CAD build for the part. Positions are in the model's coordinates, mm. Round coordinates to 2 decimals unless told otherwise and drop trailing zeros. Loops run counter-clockwise (first coordinate to the right, second up) from the corner with the lowest first, then second, coordinate; pieces in that order, holes last. Notation, with made-up numbers: M -24.75,41.5 L -8.75,41.5 A6 cw -8.75,46.5 Z; hole C 72.5,72 d10. An arc over 180 degrees is marked long. Use one line per item in the form item = value.
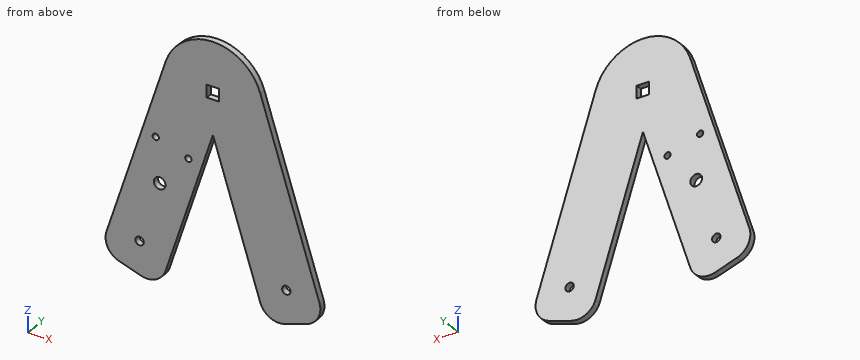
from build123d import *

# Parameters (mm, degrees)
SKETCH1_R           = 2.15
SKETCH1_R_2         = 3
SKETCH1_R_3         = 1.6
SKETCH1_W           = 6.35
SKETCH1_H           = 6.35
BOSS_EXTRUDE1_DEPTH = 3.175
FILLET1_R           = 10


with BuildPart() as part:
    # Sketch1 → Boss-Extrude1 (new body)
    with BuildSketch(Plane(origin=(0, 0, 0), x_dir=(1, 0, 0), z_dir=(0, 1, 0))):
        with BuildLine():
            Line((-57.479624947, 95.534974299), (-24.175240451, -7.792159464))
            ThreePointArc((-24.175240451, -7.792159464), (0, -25.4), (24.175240451, -7.792159464))
            Line((24.175240451, -7.792159464), (57.479624947, 95.534974299))
            Line((57.479624947, 95.534974299), (27.260574383, 105.27517363))
            Line((27.260574383, 105.27517363), (0, 20.69901171))
            Line((0, 20.69901171), (-27.260574383, 105.27517363))
            Line((-27.260574383, 105.27517363), (-57.479624947, 95.534974299))
        make_face()
        with Locations((37.5, 85.295548682)):
            Circle(SKETCH1_R, mode=Mode.SUBTRACT)
        with Locations((-37.5, 85.295548682)):
            Circle(SKETCH1_R, mode=Mode.SUBTRACT)
        with Locations((-27.222939289, 53.410881158)):
            Circle(SKETCH1_R_2, mode=Mode.SUBTRACT)
        with Locations((-29.231398698, 31.119883181)):
            Circle(SKETCH1_R_3, mode=Mode.SUBTRACT)
        with Locations((-12.575229096, 36.488496985)):
            Circle(SKETCH1_R_3, mode=Mode.SUBTRACT)
        Rectangle(SKETCH1_W, SKETCH1_H, mode=Mode.SUBTRACT)
    extrude(amount=BOSS_EXTRUDE1_DEPTH)

    # Fillet1
    fillet1_edges = [part.edges().sort_by_distance(p)[0] for p in [
        (-27.260574383, 1.5875, -105.27517363),
        (27.260574383, 1.5875, -105.27517363),
        (57.479624947, 1.5875, -95.534974299),
        (-57.479624947, 1.5875, -95.534974299),
    ]]
    fillet(fillet1_edges, radius=FILLET1_R)


solid = part.part
1. Cut at A-A on z = -70. Write the cut outline in (x, y) (3 decimals), and give its area (3 significant figures).
Completed:
outline = M -49.249,0 L -15.891,0 L -15.891,3.175 L -49.249,3.175 Z; M 15.891,0 L 49.249,0 L 49.249,3.175 L 15.891,3.175 Z
area = 212 mm2
2. Cut at B-B on y = 1.2. State how many separate pieces and enclosed holes the cut face has, and give its area (3 significant figures).
Completed:
separate_pieces = 1
enclosed_holes = 6
area = 7,380 mm2
3. Cut at C-C on x = 17. Write the cut outline in (y, z) (3 decimals), and give its area (3 significant figures).
Completed:
outline = M 0,-73.442 L 3.175,-73.442 L 3.175,18.872 L 0,18.872 Z
area = 293 mm2
4. Cut at D-D on x = -45. Write the cut outline in (y, z) (3 decimals).
Completed:
outline = M 0,-99.557 L 3.175,-99.557 L 3.175,-56.817 L 0,-56.817 Z
5. Probe line 1 along X through (y, z) = (1.9, -54); line 2 along X through (y, z) = (0.95, -55); line 3 along X through (y, z) = (1.1, -47). List the from-to ranges inside material, lowest first. Write a range as from..to.
Completed:
line_1 = -44.09..-30.16, -24.28..-10.73, 10.73..44.09
line_2 = -44.41..-29.77, -24.68..-11.06, 11.06..44.41
line_3 = -41.84..-8.48, 8.48..41.84
6. Drop flat-ended pins along their axis: P1, Ø1, axis at x = 0.5, y = 1.5, coming from the +Z side; P2, Ø1.6, axis at y = 2, z = -1.5, coming from the -X side; P3, Ø1, axis at y = 1, z = -1, coming from the +X side; P4, Ø1, axis at y = 1, z = -51.5, coming from the +X side. Give the stop position or say it passes through.
Completed:
P1 = 25.4
P2 = -27.43
P3 = 27.17
P4 = 43.45
